Study the drawing (mm; zero at the part's minimum x, y, z) and answer. A direction names the side the tool comes from. Give positions to 0.01 mm unless a question says otherwise; leave off trailing zeros. Loops run counter-clockwise (first coordinate to the right, second up) from the corner with the lowest first, then second, coordinate; pieces in that order, holes last. Notation, with made-up numbers: (72, 4.25) - (130, 4.25) arc R36 cw to (130, 39.25) - close; hole circle Ø2 at (19.5, 34). An arc over 180 degrees is marked (long way). Write item = value, one per line. Start each with the question number.
1) Consider probe 1 along Y at (x, z) = (23.5, 7.5); probe 2 along Y at (x, z) = (23.5, 2.25); probe 3 along Z at (x, y) = (42.5, 35). Determine where each line is inside the solid, lowest interval first.
2) The part is cut by section A-A on y = 23.5. Write down the section's boundary in (x, z).
3) The mould has two halves that part along X. Classify the marked faces 1, 2 and 3: +X half, -X half, draft (parallel to the pull), parting line (faces both ways), or undercut.
4) Flat-ended cylindrical pins translate along their axes: P1, Ø2, axis at x = 12.5, z = 6.5, coming from the -Y side; P2, Ø1, axis at x = 28, y = 10.5, coming from the +Z side; P3, Ø3, axis at x = 42, z = 1, coming from the +Y side (3 decimals). Find the tip coordinate at first contact, or state that the pin passes through.
5) Which of the six approach directions +Z, -Z, +X, -X, +Y, -Y give full straight-line access (tool end or side, diameter ignored) to the marked faces 4 and 5?
6) The part is cut by section D-D on y = 18. Write down the section's boundary in (x, z).
7) The part is cut by section B-B on x = 23.5. Write down the section's boundary in (y, z).
8) The part is cut by section C-C on z = 6. Write down the section's boundary in (x, y).
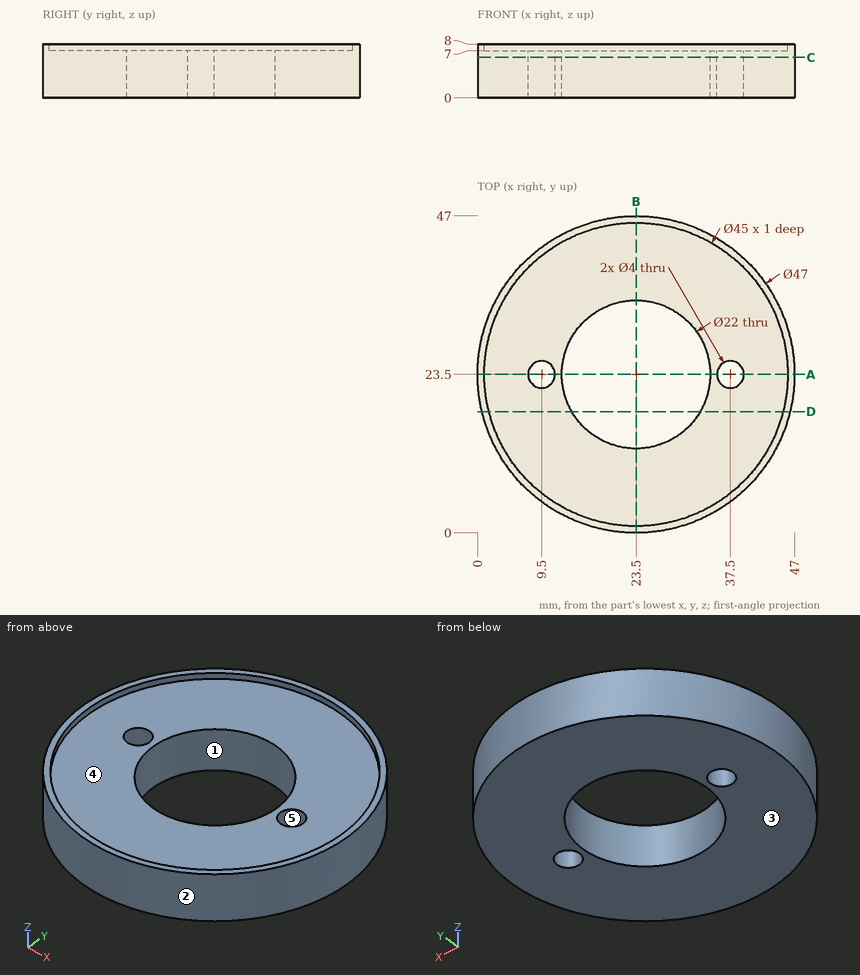
Answer below:
q1.probe_1 = 0 to 1, 46 to 47
q1.probe_2 = 0 to 12.5, 34.5 to 47
q1.probe_3 = 0 to 7
q2.outline = (0, 0) - (7.5, 0) - (7.5, 7) - (1, 7) - (1, 8) - (0, 8) - close; (11.5, 0) - (12.5, 0) - (12.5, 7) - (11.5, 7) - close; (34.5, 0) - (35.5, 0) - (35.5, 7) - (34.5, 7) - close; (39.5, 0) - (47, 0) - (47, 8) - (46, 8) - (46, 7) - (39.5, 7) - close
q3.face_1 = undercut
q3.face_2 = parting line
q3.face_3 = draft
q4.P1 = 2.23
q4.P2 = 7
q4.P3 = 39.725
q5.face_4 = +Z
q5.face_5 = +Z, -Z
q6.outline = (0.65, 0) - (13.97, 0) - (13.97, 7) - (1.68, 7) - (1.68, 8) - (0.65, 8) - close; (33.03, 0) - (46.35, 0) - (46.35, 8) - (45.32, 8) - (45.32, 7) - (33.03, 7) - close
q7.outline = (0, 0) - (12.5, 0) - (12.5, 7) - (1, 7) - (1, 8) - (0, 8) - close; (34.5, 0) - (47, 0) - (47, 8) - (46, 8) - (46, 7) - (34.5, 7) - close
q8.outline = circle Ø47 at (23.5, 23.5); hole circle Ø4 at (9.5, 23.5); hole circle Ø22 at (23.5, 23.5); hole circle Ø4 at (37.5, 23.5)
